from build123d import *

# Parameters (mm, degrees)
SKETCH1_R             = 30
BOSS_EXTRUDE1_DEPTH   = 15
CUT_EXTRUDE1_REACH    = 47
SKETCH2_R             = 9.765
SKETCH3_R             = 12.5
CUT_EXTRUDE2_DEPTH    = 5
FILLET1_R             = 1
M6_TAPPED_HOLE1_D     = 5
M6_TAPPED_HOLE1_DEPTH = 17
M6_TAPPED_HOLE1_TIP   = 1.502151548
F_8_0MM_DOWEL_HOLE1_D = 8


with BuildPart() as part:
    # Sketch1 → Boss-Extrude1 (new body)
    with BuildSketch(Plane(origin=(0, 0, 0), x_dir=(1, 0, 0), z_dir=(0, 1, 0))):
        with Locations(Location((0, 0, 0), (0, 0, 270))):
            Circle(SKETCH1_R)
    extrude(amount=BOSS_EXTRUDE1_DEPTH)

    # Sketch2 → Cut-Extrude1 (cut, up to next)
    with BuildSketch(Plane(origin=(0, 15, 0), x_dir=(1, 0, 0), z_dir=(0, 1, 0)), mode=Mode.PRIVATE) as cut_extrude1_sk1:
        with Locations(Location((0, 0, 0), (0, 0, 270))):
            Circle(SKETCH2_R)
    cut_extrude1_tool1 = extrude(cut_extrude1_sk1.sketch, amount=-CUT_EXTRUDE1_REACH, mode=Mode.PRIVATE) & part.part
    add(cut_extrude1_tool1.solids().sort_by_distance((0, 15, 0))[0], mode=Mode.SUBTRACT)

    # Sketch3 → Cut-Extrude2 (cut)
    with BuildSketch(Plane(origin=(0, 15, 0), x_dir=(1, 0, 0), z_dir=(0, 1, 0))):
        with Locations(Location((0, 0, 0), (0, 0, 270))):
            Circle(SKETCH3_R)
    extrude(amount=-CUT_EXTRUDE2_DEPTH, mode=Mode.SUBTRACT)

    # Fillet1
    fillet1_edges = [part.edges().sort_by_distance(p)[0] for p in [
        (0, 10, -9.765),
    ]]
    fillet(fillet1_edges, radius=FILLET1_R)

    # M6 Tapped Hole1
    with Locations(Plane(origin=(0, 15, 0), x_dir=(1, 0, 0), z_dir=(0, 1, 0))):
        with Locations((0, 22.5), (19.485571585, -11.25), (-19.485571585, -11.25)):
            Hole(M6_TAPPED_HOLE1_D / 2, depth=M6_TAPPED_HOLE1_DEPTH)
            with Locations((0, 0, -(M6_TAPPED_HOLE1_DEPTH + M6_TAPPED_HOLE1_TIP / 2))):  # 118° drill point
                Cone(0, M6_TAPPED_HOLE1_D / 2, M6_TAPPED_HOLE1_TIP, mode=Mode.SUBTRACT)

    # Ø8.0mm Dowel Hole1 (through all)
    with Locations(Plane(origin=(0, 15, 0), x_dir=(1, 0, 0), z_dir=(0, 1, 0))):
        with Locations((22.5, 0), (-22.5, 0)):
            Hole(F_8_0MM_DOWEL_HOLE1_D / 2)


solid = part.part
Geometry: final body of the model. Coordinates: model frame, mm. A direction names the side the tool comes from. Coordinates: 2 decimals unless noted, no trailing zeros. Order: outer loops, then holes, each group sorted by start corner. A loop starts at its lowest first (then second) coordinate and runs counter-clockwise, first axis right, second up. Notation, with made-up numbers: (56, 37) - (92, 37) arc R30 ccw to (92, 68) - close; hole circle Ø7 at (-16.5, 11.5). An arc over 180 degrees is marked (long way). Use one line per item in the form item = value.
1) Mould query, pull axis Z, two halves, no side actions, for faces 1 (the face through (0, 15, 13)), 2 (the face through (-20.639, 7.395, 13.468)), 3 (the face through (1.32, 7.4, -29.97)). Classes: +Z half, -Z half, draft (parallel to the pull), parting line (faces both ways), or undercut.
Solutions:
face_1 = draft
face_2 = undercut
face_3 = parting line
2) Section D-D (x = -23). Return loops of the section in (y, z), then the cut area to 3 significant figures.
Solutions:
outline = (0, -19.26) - (15, -19.26) - (15, -3.97) - (0, -3.97) - close; (0, 3.97) - (15, 3.97) - (15, 19.26) - (0, 19.26) - close
area = 459 mm^2
3) Ray query, L1, parallel to X at y = 9.75, z = 11.25; L2, parallel to X at y = 13.75, z = 2.5; L3, parallel to Z at x = -1, y = 5.75. Return the intervals inside material, ascending.
Solutions:
L1 = -27.81 to -21.99, -16.99 to 16.99, 21.99 to 27.81
L2 = -29.9 to -25.62, -19.38 to -12.25, 12.25 to 19.38, 25.62 to 29.9
L3 = -29.98 to -24.79, -20.21 to -9.71, 9.71 to 29.98
4) Pin query (flat end, axial travel): pin 1 (2 mm diameter, centred on y = 3, z = 18, fed in from -X); pin 2 (1.5 mm diameter, centred on x = -13.5, y = 4.5, fed in from -Z); pin 3 (8 mm diameter, centred on y = 2.5, z = 8, fed in from +X); pin 4 (3 mm diameter, centred on x = -19.49, z = 11.25, fed in from +Y). Return the tip coordinate at first contact, or that it passes through.
Solutions:
pin_1 = -24.72
pin_2 = -27.16
pin_3 = 29.73
pin_4 = through
5) Set-up query: faces 4 (the face through (25.7, 7.4, 2.4)), 5 (the face through (3.755, 12.535, 11.923)). Return all of +Z, -Z, +X, -X, +Y, -Y with unobstructed straight access to the full face (end or side cutting, diameter ignored); none if empty.
Solutions:
face_4 = +Y, -Y
face_5 = +Y
6) Section C-C (x = 0). Return loops of the section in (y, z) (3 decimals), then the cut area to 3 significant figures.
Solutions:
outline = (0, -30) - (15, -30) - (15, -25) - (0, -25) - close; (0, -20) - (15, -20) - (15, -12.5) - (10, -12.5) - (10, -10.765) arc R1 ccw to (9, -9.765) - (0, -9.765) - close; (0, 9.765) - (9, 9.765) arc R1 ccw to (10, 10.765) - (10, 12.5) - (15, 12.5) - (15, 30) - (0, 30) - close
area = 504 mm^2
7) Section B-B (z = 0). Return loops of the section in (x, y) (3 decimals).
Solutions:
outline = (-30, 0) - (-26.5, 0) - (-26.5, 15) - (-30, 15) - close; (-18.5, 0) - (-9.765, 0) - (-9.765, 9) arc R1 ccw to (-10.765, 10) - (-12.5, 10) - (-12.5, 15) - (-18.5, 15) - close; (9.765, 0) - (18.5, 0) - (18.5, 15) - (12.5, 15) - (12.5, 10) - (10.765, 10) arc R1 ccw to (9.765, 9) - close; (26.5, 0) - (30, 0) - (30, 15) - (26.5, 15) - close
8) Section A-A (y = 14.25). Return loops of the section in (x, z), then the cut area to 3 significant figures.
Solutions:
outline = circle Ø60 at (0, 0); hole circle Ø8 at (-22.5, 0); hole circle Ø5 at (-19.49, 11.25); hole circle Ø25 at (0, 0); hole circle Ø5 at (0, -22.5); hole circle Ø5 at (19.49, 11.25); hole circle Ø8 at (22.5, 0)
area = 2,180 mm^2
